```python
from build123d import *

# Parameters (mm, degrees)
F1_DEPTH = 17
F2_W     = 6.5
F2_H     = 9
F3_DEPTH = 25


with BuildPart() as f1:
    # F0 (on Top) → F1 (new body)
    with BuildSketch(Plane.XY):
        Polygon((-15.092822, 2.267766), (-12.592822, -0.232234), (7.407178, -0.232234), (7.407178, -21.232234), (-12.592822, -21.232234), (-15.092822, -23.732234), (9.907178, -23.732234), (9.907178, 2.267766), align=None)
    extrude(amount=F1_DEPTH)

    # F2 (on face) → F3 (cut)
    with BuildSketch(Plane.YZ.offset(9.907178)):
        with Locations((-10.732234, 12.5)):
            Rectangle(F2_W, F2_H)
    extrude(amount=-F3_DEPTH, mode=Mode.SUBTRACT)


solid = f1.part
```
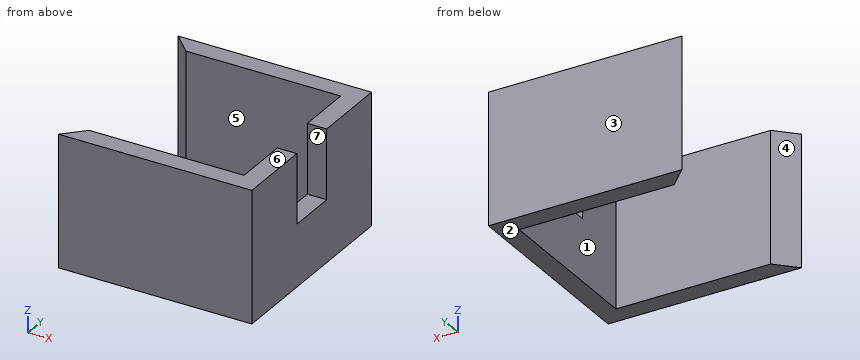
Verification items for the finished model (mm, model axes). Face numbers are marked on the shaded views. A direction names the side the tool comes from. Coordinates: 2 decimals unless noted, no trailing zeros. Order: outer loops, then holes, each group sorted by start corner. A loop starts at its lowest first (then second) coordinate and runs counter-clockwise, first axis right, second up. Notation, with made-up numbers: (56.5, 34) - (65.5, 34) arc R30 ccw to (65.5, 66) - close; hole circle Ø10 at (71, 82). An arc over 180 degrees is marked (long way). Return JSON: item names as keys, results as strings.
(1) Section check D-D, the plane y = -3.25. Record the cut outline in (x, z), and give its area (3 significant figures).
Filled sheet:
{"outline": "(7.41, 0) - (9.91, 0) - (9.91, 17) - (7.41, 17) - close", "area": "42.5 mm^2"}
(2) Section check C-C, the plane y = -12.25. Record the cut outline in (x, z).
Filled sheet:
{"outline": "(7.41, 0) - (9.91, 0) - (9.91, 8) - (7.41, 8) - close"}
(3) Go/stop test with flat-tipped pins: pin 1 (4 mm diameter, centred on y = -17.5, z = 3.5, fed in from -X); pin 2 (3 mm diameter, centred on x = 8, y = -10.5, fed in from +Z). Record where each tip stops, or that it passes through.
Filled sheet:
{"pin 1": "stops at x = 7.41", "pin 2": "stops at z = 8"}
(4) Mould release check, pull along Y, two halves, no side actions. Record for the marked faces 1, 2, 3 and 4: pulls with the +Y half, pulls with the -Y half, needs draft (parallel to the pull), parting line crosses it, or undercut.
Filled sheet:
{"face 1": "undercut", "face 2": "needs draft", "face 3": "pulls with the +Y half", "face 4": "undercut"}
(5) Section check A-A, the plane z = 15. Record the cut outline in (x, y), and give its area (3 significant figures).
Filled sheet:
{"outline": "(-15.09, -23.73) - (9.91, -23.73) - (9.91, -13.98) - (7.41, -13.98) - (7.41, -21.23) - (-12.59, -21.23) - close; (-15.09, 2.27) - (-12.59, -0.23) - (7.41, -0.23) - (7.41, -7.48) - (9.91, -7.48) - (9.91, 2.27) - close", "area": "155 mm^2"}
(6) Section check B-B, the plane x = -4.5. Record the cut outline in (y, z).
Filled sheet:
{"outline": "(-23.73, 0) - (-21.23, 0) - (-21.23, 17) - (-23.73, 17) - close; (-0.23, 0) - (2.27, 0) - (2.27, 17) - (-0.23, 17) - close"}
(7) Access from +Z, -Z, +X, -X, +Y, -Y to the whole of each face (thin tool, end or side, straight path). Record for the marked faces 5, 6 and 7.
Filled sheet:
{"face 5": "+Z, -Z, -X", "face 6": "+Z, +X, -X, +Y, -Y", "face 7": "+Z, +X, -X"}
(8) Thickness scan on line 1 along Y through (x, z) = (7.5, 13.75); line 2 along Y through (x, z) = (1.75, 6.5); line 3 along X through (y, z) = (-9.5, 3.75). Record the ranges inside material, lowest first.
Filled sheet:
{"line 1": "y = -23.73 to -13.98, -7.48 to 2.27", "line 2": "y = -23.73 to -21.23, -0.23 to 2.27", "line 3": "x = 7.41 to 9.91"}
